Here's how the part is built. I have some questions about the finished solid (model axes, mm). A direction names the side the tool comes from. Coordinates: 2 decimals unless noted, no trailing zeros. Write each loop counter-clockwise with the first axis right and the second up, starting at its lowest first coordinate (ties: lowest second). Pieces come first, ordered by that corner, then holes. Notation, with made-up numbers: (87.5, 38) - (133.5, 38) arc R28 ccw to (133.5, 76) - close; hole circle Ø8 at (60.5, 26.5). An arc over 180 degrees is marked (long way). Answer in a Markdown table with one row per item. Add a question column.
Item 1: I'm going to push flat-ended pins straight in: pin 1 (10 mm diameter, centred on x = -32.5, z = 5.5, fed in from +Y); pin 2 (13 mm diameter, centred on x = 0, y = 0, fed in from -Z); pin 3 (10 mm diameter, centred on x = -30.5, z = 6.5, fed in from -Y). Where does each tip first touch, or does it pass through?
Item 2: We'd pull the mould along Y, two halves only. Please class faces 1 (the face through (3.22, 24.54, -10.37)), 2 (the face through (-23, 45, 11.85)): +Y half, -Y half, draft (parallel to the pull), parting line (faces both ways), or undercut.
Item 3: If I drill on probe 1 along Y at (x, z) = (0, 10.75); probe 2 along Y at (x, z) = (0, -9.85); probe 3 along Y at (x, z) = (0, -2.5), over which ranges is the centre line in solid material (lowest first)? Write a range as from..to.
Item 4: Imagine slicing it at D-D (y = -30). Please give me the cut outline in (x, z), plus the area to 3 significant figures.
Item 5: Imagine slicing it at A-A (y = 0). Please give me the cut outline in (x, z).
Item 6: Which directions (+Z, -Z, +X, -X, +Y, -Y) give clear straight access to the entire face, cutting with the end or side of a thin tool? Please do faces 3 (the face through (9, 1, 11.85)), 4 (the face through (-9, -40, 11)), 5 (the face through (-5.2, 0.3, -8.85)).
Item 7: Imagine slicing it at C-C (z = 4.25). Please give me the cut outline in (x, y).
from build123d import *

# Parameters (mm, degrees)
SKETCH1_R           = 60
SKETCH1_R_2         = 50
SKETCH1_R_3         = 41
SKETCH1_R_4         = 5
BOSS_EXTRUDE1_DEPTH = 11.85
SKETCH2_R           = 50
SKETCH2_R_2         = 41
CUT_EXTRUDE1_DEPTH  = 1.6
SKETCH3_R           = 24.75
CUT_EXTRUDE2_DEPTH  = 3


with BuildPart() as part:
    # Sketch1 → Boss-Extrude1 (new, symmetric)
    # profile 1 of 3: a face of its own
    with BuildSketch(Plane.XY):
        Circle(SKETCH1_R)
        Circle(SKETCH1_R_2, mode=Mode.SUBTRACT)
    # profile 2 of 3: a face of its own
    with BuildSketch(Plane.XY):
        Circle(SKETCH1_R_2)
        Circle(SKETCH1_R_3, mode=Mode.SUBTRACT)
    # profile 3 of 3: a face of its own
    with BuildSketch(Plane.XY):
        Circle(SKETCH1_R_3)
        Circle(SKETCH1_R_4, mode=Mode.SUBTRACT)
    extrude(amount=BOSS_EXTRUDE1_DEPTH, both=True)

    # Sketch2 → Cut-Extrude1 (cut)
    with BuildSketch(Plane.XY.offset(11.85)):
        Circle(SKETCH2_R)
        Circle(SKETCH2_R_2, mode=Mode.SUBTRACT)
    extrude(amount=-CUT_EXTRUDE1_DEPTH, mode=Mode.SUBTRACT)

    # Sketch3 → Cut-Extrude2 (cut)
    with BuildSketch(Plane(origin=(0, 0, -11.85), x_dir=(-1, 0, 0), z_dir=(0, 0, -1))):
        Circle(SKETCH3_R)
    extrude(amount=-CUT_EXTRUDE2_DEPTH, mode=Mode.SUBTRACT)


solid = part.part
Here are the results:
| question | item | result |
|---|---|---|
| 1 | pin 1 | stops at y = 53.33 |
| 1 | pin 2 | stops at z = -8.85 |
| 1 | pin 3 | stops at y = -54.31 |
| 2 | face 1 | undercut |
| 2 | face 2 | draft |
| 3 | probe 1 | y = -60..-50, -41..-5, 5..41, 50..60 |
| 3 | probe 2 | y = -60..-24.75, 24.75..60 |
| 3 | probe 3 | y = -60..-5, 5..60 |
| 4 | outline | (-51.96, -11.85) - (51.96, -11.85) - (51.96, 11.85) - (40, 11.85) - (40, 10.25) - (27.95, 10.25) - (27.95, 11.85) - (-27.95, 11.85) - (-27.95, 10.25) - (-40, 10.25) - (-40, 11.85) - (-51.96, 11.85) - close |
| 4 | area | 2,420 mm2 |
| 5 | outline | (-60, -11.85) - (-24.75, -11.85) - (-24.75, -8.85) - (-5, -8.85) - (-5, 11.85) - (-41, 11.85) - (-41, 10.25) - (-50, 10.25) - (-50, 11.85) - (-60, 11.85) - close; (5, -8.85) - (24.75, -8.85) - (24.75, -11.85) - (60, -11.85) - (60, 11.85) - (50, 11.85) - (50, 10.25) - (41, 10.25) - (41, 11.85) - (5, 11.85) - close |
| 6 | face 3 | +Z, +X, -X, +Y, -Y |
| 6 | face 4 | +Z |
| 6 | face 5 | -Z |
| 7 | outline | circle Ø120 at (0, 0); hole circle Ø10 at (0, 0) |
